from build123d import *

# Parameters (mm, degrees)
F1_ANGLE = 270
F14_T    = -3
F3_D     = 3
F5_D     = 3
F7_ANGLE = 135
F9_D     = 3
F11_D    = 3
F13_D    = 3


with BuildPart() as f1:
    # F0 (on Top) → F1 (revolve)
    with BuildSketch(Plane.XY):
        with BuildLine():
            ThreePointArc((15, 0), (0, 15), (-15, 0))
            Line((-15, 0), (15, 0))
        make_face()
    revolve(axis=Axis((0.571103, 0, 0), (1, 0, 0)), revolution_arc=F1_ANGLE)

    # F14
    f14_openings = [f1.faces().sort_by_distance(p)[0] for p in [
        (0, 6.366198, 0),
        (0, 0, -6.366198),
    ]]
    offset(amount=F14_T, openings=f14_openings)

    # F3 (through all)
    with Locations(Plane.YZ):
        with Locations((0, 0)):
            Hole(F3_D / 2)

    # F5 (through all)
    with Locations(Plane(origin=(0, 0, 0), x_dir=(0, 1, 0), z_dir=(-1, 0, 0))):
        with Locations((0, 0)):
            Hole(F5_D / 2)


with BuildPart() as f1_1:
    # F7: moved
    add(f1.part.rotate(Axis((0, 0, 0), (-1, 0, 0)), F7_ANGLE))

    # F9 (through all)
    with Locations(Plane.XZ):
        with Locations((0, 0)):
            Hole(F9_D / 2)

    # F11 (through all)
    with Locations(Plane.XY):
        with Locations((0, 0)):
            Hole(F11_D / 2)

    # F13 (through all)
    with Locations(Plane(origin=(0, 0, 0), x_dir=(1, 0, 0), z_dir=(0, 0, -1))):
        with Locations((0, 0)):
            Hole(F13_D / 2)


solid = f1_1.part
For this review, take the finished solid that the model builds, in its own axes (mm). Give positions to 0.01 mm unless a question says otherwise; leave off trailing zeros. Order: outer loops, then holes, each group sorted by start corner. A loop starts at its lowest first (then second) coordinate and runs counter-clockwise, first axis right, second up. Notation, with made-up numbers: M 16,68.25 L 46,68.25 A24 ccw 46,89.25 Z; hole C 52.5,51.5 d4. An arc over 180 degrees is marked long. Answer in a Markdown table with one row per item. Add a question column.
(1) Mouldability with a two-part tool opening along Z and no side actions: class faces 1 (the face through (1.5, 0.07, -13.44)), 2 (the face through (1, -9, 9)), 3 (the face through (1, -9, -9)) as +Z half, -Z half, draft (parallel to the pull), parting line (faces both ways), or undercut.
(2) Consider section D-D on y = -2.75. State the section outline as (x, z) points.
(3) Wall thickness on probe 1 along X at (y, z) = (0.25, 5); probe 2 along X at (y, z) = (-2, -3.5); probe 3 along Z at (x, y) = (13.45, 0): over which ranges is each line inside the solid? List them lowest first. Write a range as [from, to].
(4) Consider section B-B on z = 0. State the section outline as (x, y) points, and give its area (3 significant figures).
(5) For pin 1 (1.8 mm diameter, centred on y = 0, z = 0, fed in from +X); pin 2 (4 mm diameter, centred on x = -2.5, z = -3, fed in from -Y); pin 3 (2 mm diameter, centred on x = -2, z = -9.5, fed in from +Y); pin 4 (1.5 mm diameter, centred on x = 7, z = -11, fed in from +Y), all flat-tipped, find the tip position at first contact; note any pin that passes through.
(6) Consider section A-A on y = 0. State the section outline as (x, z) points, and give its area (3 significant figures).
(7) Consider section C-C on x = 0. State the section outline as (y, z) points.
Evaluation:
| question | item | result |
|---|---|---|
| 1 | face 1 | draft |
| 1 | face 2 | undercut |
| 1 | face 3 | undercut |
| 2 | outline | M -14.49,-2.75 A14.75 ccw 14.49,-2.75 L 11.35,-2.75 A11.68 cw -11.35,-2.75 Z; M -14.49,2.75 L -11.35,2.75 A11.68 cw 11.35,2.75 L 14.49,2.75 A14.75 ccw Z |
| 3 | probe 1 | x = [-14.14, -10.91], [10.91, 14.14] |
| 3 | probe 2 | x = [-14.45, -11.3], [11.3, 14.45] |
| 3 | probe 3 | z = [-6.64, -1.5], [1.5, 6.64] |
| 4 | outline | M -14.92,1.5 L -11.91,1.5 A12 cw -1.5,11.91 L -1.5,14.92 A15 ccw Z; M 1.5,11.91 A12 cw 11.91,1.5 L 14.92,1.5 A15 ccw 1.5,14.92 Z |
| 4 | area | 109 mm^2 |
| 5 | pin 1 | passes through |
| 5 | pin 2 | stops at y = 10.45 |
| 5 | pin 3 | stops at y = 12.21 |
| 5 | pin 4 | stops at y = 8.6 |
| 6 | outline | M -14.92,-1.5 A15 ccw -1.5,-14.92 L -1.5,-11.91 A12 cw -11.91,-1.5 Z; M -14.92,1.5 L -11.91,1.5 A12 cw -1.5,11.91 L -1.5,14.92 A15 ccw Z; M 1.5,-14.92 A15 ccw 14.92,-1.5 L 11.91,-1.5 A12 cw 1.5,-11.91 Z; M 1.5,11.91 A12 cw 11.91,1.5 L 14.92,1.5 A15 ccw 1.5,14.92 Z |
| 6 | area | 218 mm^2 |
| 7 | outline | M -10.61,-10.61 A15 ccw -1.5,-14.92 L -1.5,-11.91 A12 cw -8.49,-8.49 Z; M -10.61,10.61 L -8.49,8.49 A12 cw -1.5,11.91 L -1.5,14.92 A15 ccw Z; M 1.5,-14.92 A15 ccw 14.92,-1.5 L 11.91,-1.5 A12 cw 1.5,-11.91 Z; M 1.5,11.91 A12 cw 11.91,1.5 L 14.92,1.5 A15 ccw 1.5,14.92 Z |
